Check sheet for the drawn part. Datum: minimum x, y, z corner. Units: mm. A direction names the side the tool comes from. Give positions to 0.01 mm unless a question says otherwise; leave off trailing zeros. Write each loop counter-clockwise with the first axis right and the second up, starting at its lowest first coordinate (ties: lowest second). Pieces come first, ordered by that corner, then holes.
(1) Cross-section at C-C (z = 17.5). Record the boundary of the cut face in (x, y), and give its area (3 significant figures).
(2) Tool access check on the marked faces 5, 6 and 7. Record the directions out of +Z, -Z, +X, -X, +Y, -Y that give a thin tool (end or side, any length) a straight path to the whole face; none if there is none.
(3) Depth check by flat-ended pin: P1, Ø1, axis at x = 13.5, z = 9.5, coming from the -Y side; P2, Ø5, axis at y = 10, z = 17.5, coming from the -X side; P3, Ø5, axis at x = 2, y = 34.5, coming from the -Z side; P4, Ø8, axis at x = 6, z = 16.5, coming from the -Y side. Enter the tip coordinate at first touch or a pass-through.
(4) Thickness scan on line 1 along Y through (x, z) = (13.55, 11); line 2 along X through (y, z) = (5.5, 8.5); line 3 along Z through (x, y) = (14.15, 31). Record the ranges inside material, lowest first.
(5) Cross-section at D-D (x = 10). Record the boundary of the cut face in (y, z).
(6) Cross-section at B-B (x = 4.5). Record the boundary of the cut face in (y, z), and give its area (3 significant figures).
(7) Cross-section at A-A (y = 10). Record the boundary of the cut face in (x, z).
(8) Mould release check, pull along Z, two halves, no side actions. Record for the marked faces 1, 2, 3 and 4: +Z half, -Z half, draft (parallel to the pull), parting line (faces both ways), or undercut.
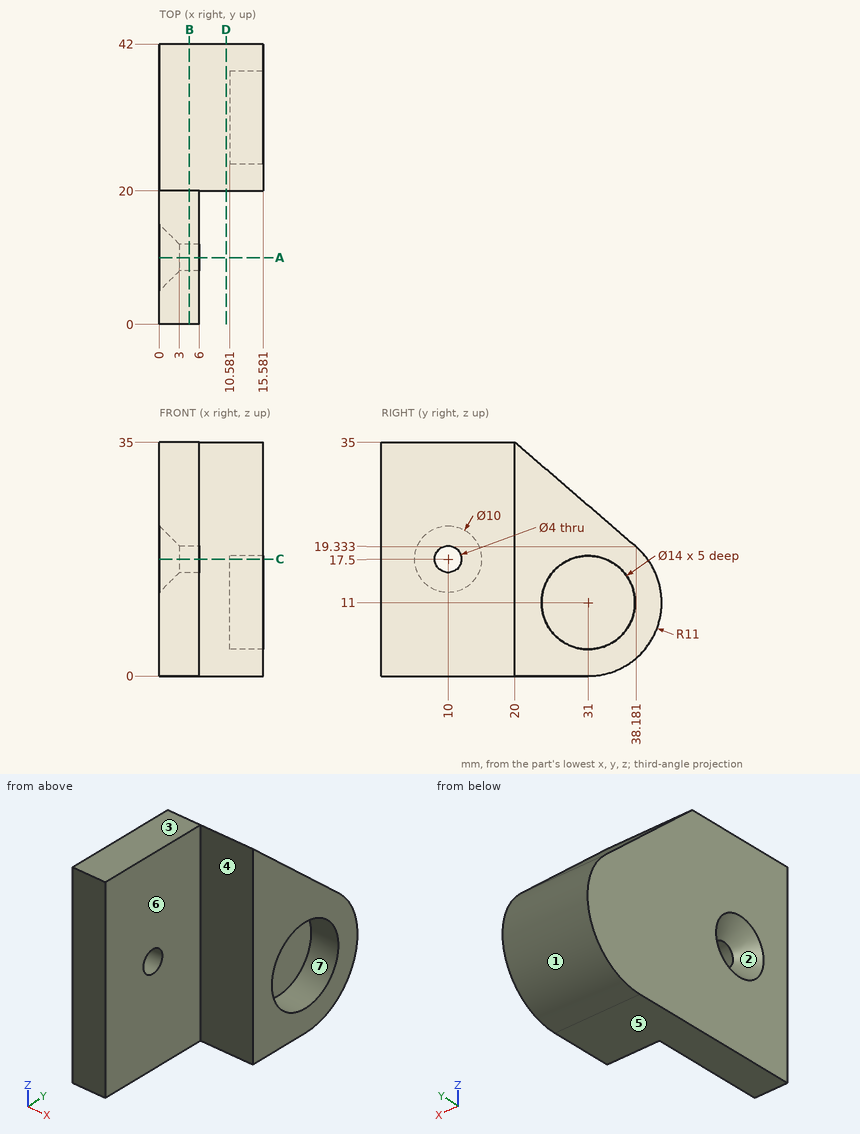
Reply:
1. outline: (0, 0) - (6, 0) - (6, 8) - (3, 8) - (0, 5) - close; (0, 15) - (3, 12) - (6, 12) - (6, 20) - (15.58, 20) - (15.58, 28.4) - (10.58, 28.4) - (10.58, 33.6) - (15.58, 33.6) - (15.58, 39.87) - (0, 39.87) - close
1. area: 371 mm2
2. face 5: -Z, +X, -X, +Y, -Y
2. face 6: +Z, -Z, +X, -Y
2. face 7: +X
3. P1: stops at y = 20
3. P2: stops at x = 2.5
3. P3: stops at z = 0.05
3. P4: stops at y = 0
4. line 1: y = 20 to 24, 38 to 42
4. line 2: x = 0 to 6
4. line 3: z = 0 to 4, 18 to 25.52
5. outline: (20, 0) - (31, 0) arc R11 ccw to (38.18, 19.33) - (20, 35) - close
6. outline: (0, 0) - (31, 0) arc R11 ccw to (38.18, 19.33) - (20, 35) - (0, 35) - close; hole circle Ø4 at (10, 17.5)
6. area: 1,220 mm2
7. outline: (0, 0) - (6, 0) - (6, 15.5) - (3, 15.5) - (0, 12.5) - close; (0, 22.5) - (3, 19.5) - (6, 19.5) - (6, 35) - (0, 35) - close
8. face 1: parting line
8. face 2: undercut
8. face 3: +Z half
8. face 4: draft
